from build123d import *

# Parameters (mm, degrees)
F1_DEPTH = 45
F2_W     = 10
F2_H     = 3
F3_DEPTH = 25
F4_W     = 10
F4_H     = 3
F5_DEPTH = 25


with BuildPart() as f1:
    # F0 (on Front) → F1 (new body)
    with BuildSketch(Plane.XZ):
        Polygon((79.9, 3), (0, 3), (0, -37), (3, -37), (3, 0), (76.9, 0), (76.9, -37), (79.9, -37), align=None)
    extrude(amount=F1_DEPTH)

    # F2 (on face) → F3 (cut)
    with BuildSketch(Plane.YZ.offset(79.9)):
        with Locations((-32.5, -35.5)):
            Rectangle(F2_W, F2_H)
        with Locations((-12.5, -35.5)):
            Rectangle(F2_W, F2_H)
    extrude(amount=-F3_DEPTH, mode=Mode.SUBTRACT)

    # F4 (on face) → F5 (cut)
    with BuildSketch(Plane(origin=(0, 0, 0), x_dir=(0, -1, 0), z_dir=(-1, 0, 0))):
        with Locations((12.5, -35.5)):
            Rectangle(F4_W, F4_H)
        with Locations((32.5, -35.5)):
            Rectangle(F4_W, F4_H)
    extrude(amount=-F5_DEPTH, mode=Mode.SUBTRACT)


solid = f1.part
Work out the finished part from the listing and answer in its coordinate system (mm). A direction names the side the tool comes from. Round coordinates to 2 decimals unless told otherwise and drop trailing zeros. Write each loop counter-clockwise with the first axis right and the second up, starting at its lowest first coordinate (ties: lowest second). Pieces come first, ordered by that corner, then holes. Notation, with made-up numbers: M 81,-23 L 102,-23 A21 ccw 102,-10 Z; hole C 67,-6.5 d7. An arc over 180 degrees is marked long. Use a Markdown table: item, result.
1) The part is cut by section A-A on z = -22. Give the vertices of the cut face in (x, y).
Taken from the geometry:
| item | result |
|---|---|
| outline | M 0,-45 L 3,-45 L 3,0 L 0,0 Z; M 76.9,-45 L 79.9,-45 L 79.9,0 L 76.9,0 Z |
2) The part is cut by section C-C on x = 5. Give the vertices of the cut face in (y, z), plus the area to 3 significant figures.
Taken from the geometry:
| item | result |
|---|---|
| outline | M -45,0 L 0,0 L 0,3 L -45,3 Z |
| area | 135 mm2 |
3) Determine the mould class of faces 4 (the face through (78, -22, -37)), 5 (the face through (39, -22, 0)), 6 (the face through (0, -22, -17)), 7 (the face through (79.9, -22, -17)) for opening direction X: pulls with the +X half, pulls with the -X half, needs draft (parallel to the pull), parting line crosses it, or undercut.
Taken from the geometry:
| item | result |
|---|---|
| face 4 | needs draft |
| face 5 | undercut |
| face 6 | pulls with the -X half |
| face 7 | pulls with the +X half |
4) The part is cut by section B-B on y = -34. Give the vertices of the cut face in (x, z), plus the area to 3 significant figures.
Taken from the geometry:
| item | result |
|---|---|
| outline | M 0,-34 L 3,-34 L 3,0 L 76.9,0 L 76.9,-34 L 79.9,-34 L 79.9,3 L 0,3 Z |
| area | 444 mm2 |
5) The part is cut by section D-D on y = -39. Give the vertices of the cut face in (x, z).
Taken from the geometry:
| item | result |
|---|---|
| outline | M 0,-37 L 3,-37 L 3,0 L 76.9,0 L 76.9,-37 L 79.9,-37 L 79.9,3 L 0,3 Z |
6) Consider line 1 (X direction, y = -37, z = -32); line 2 (Z direction, x = 33.5, y = -27.5). Determine where each line is inside the solid, lowest interval first. Write a range as [from, to].
Taken from the geometry:
| item | result |
|---|---|
| line 1 | x = [0, 3], [76.9, 79.9] |
| line 2 | z = [0, 3] |
7) Which of the six approach directions +Z, -Z, +X, -X, +Y, -Y give full straight-line access (tool end or side, diameter ignored) to faces 1 (the face through (78, -4, -37)), 2 (the face through (1, -32, -34)), 3 (the face through (3, -22, -19))?
Taken from the geometry:
| item | result |
|---|---|
| face 1 | -Z, +X, -X, +Y, -Y |
| face 2 | -Z, +X, -X |
| face 3 | -Z, +Y, -Y |
8) Flat-ended cylindrical pins translate along their axes: pin 1 (3.5 mm diameter, centred on x = 77.5, y = -33.5, fed in from -Z); pin 2 (10 mm diameter, centred on x = 38, y = -6.5, fed in from -Z). Find the tip coordinate at first contact, or state that the pin passes through.
Taken from the geometry:
| item | result |
|---|---|
| pin 1 | stops at z = -34 |
| pin 2 | stops at z = 0 |
